Here's the drawing with two shaded views (mm, measured from the low corner). I have some questions. A direction names the side the tool comes from. Give positions to 0.01 mm unless a question says otherwise; leave off trailing zeros. Write each loop counter-clockwise with the first axis right and the second up, starting at its lowest first coordinate (ties: lowest second). Pieces come first, ordered by that corner, then holes. Notation, with made-up numbers: (-23, 8.25) - (26, 8.25) arc R22 cw to (26, 31.25) - close; hole circle Ø7 at (0.5, -33.5). An arc over 180 degrees is marked (long way). Write item = value, one per line.
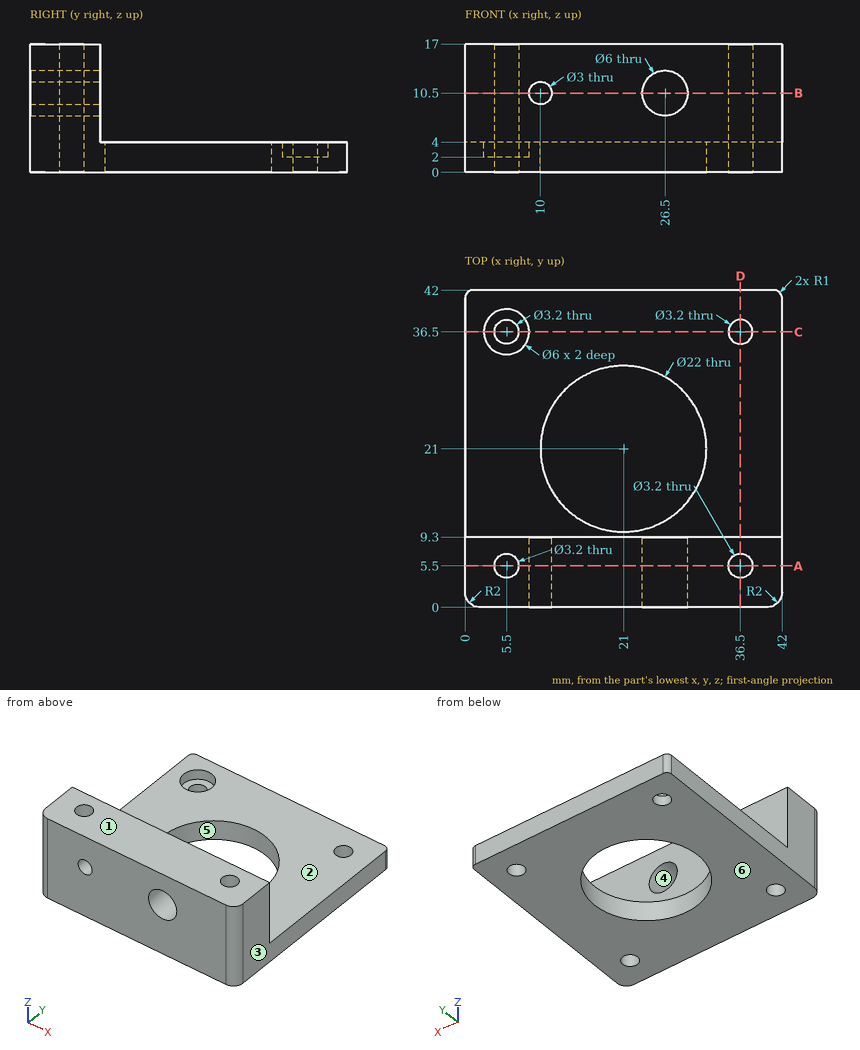
1. For pin 1 (2.5 mm diameter, centred on x = 10, z = 10.5, fed in from -Y); pin 2 (2 mm diameter, centred on x = 31, y = 31, fed in from +Z); pin 3 (4 mm diameter, centred on x = 26.5, z = 7.5, fed in from +Y); pin 4 (5 mm diameter, centred on x = 5.5, y = 36.5, fed in from +Z), each with a flat end and sliding along its axis, tell me the tip position at first contact or that it passes through.
Filled sheet:
pin_1 = through
pin_2 = 4
pin_3 = 9.3
pin_4 = 2
2. Thinking about a two-plate mould opening in X: for the marked faces 3, 4, 5 and 6, which applies, pulls with the +X half, pulls with the -X half, needs draft (parallel to the pull), parting line crosses it, or undercut?
Filled sheet:
face_3 = pulls with the +X half
face_4 = undercut
face_5 = undercut
face_6 = needs draft
3. If we section it at C-C, the plane y = 36.5: Please give me the cut outline in (x, z).
Filled sheet:
outline = (0, 0) - (3.9, 0) - (3.9, 2) - (2.5, 2) - (2.5, 4) - (0, 4) - close; (7.1, 0) - (34.9, 0) - (34.9, 4) - (8.5, 4) - (8.5, 2) - (7.1, 2) - close; (38.1, 0) - (42, 0) - (42, 4) - (38.1, 4) - close
4. Which directions (+Z, -Z, +X, -X, +Y, -Y) give clear straight access to the entire face, cutting with the end or side of a thin tool? Please do the marked faces 1 and 2.
Filled sheet:
face_1 = +Z, +X, -X, +Y, -Y
face_2 = +Z, +X, -X, +Y
5. If we section it at A-A, the plane y = 5.5: Please give me the cut outline in (x, z).
Filled sheet:
outline = (0, 0) - (3.9, 0) - (3.9, 17) - (0, 17) - close; (7.1, 0) - (34.9, 0) - (34.9, 17) - (7.1, 17) - close; (38.1, 0) - (42, 0) - (42, 17) - (38.1, 17) - close; hole circle Ø3 at (10, 10.5); hole circle Ø6 at (26.5, 10.5)
6. If we section it at D-D, the plane x = 36.5: Please give me the cut outline in (y, z), and give its area (3 significant figures).
Filled sheet:
outline = (0, 0) - (3.9, 0) - (3.9, 17) - (0, 17) - close; (7.1, 0) - (34.9, 0) - (34.9, 4) - (9.3, 4) - (9.3, 17) - (7.1, 17) - close; (38.1, 0) - (42, 0) - (42, 4) - (38.1, 4) - close
area = 222 mm2
7. I need wall thicknesses on line 1 (Y direction, x = 5.5, z = 1.4); line 2 (Y direction, x = 26.5, z = 5.5); line 3 (X direction, y = 8, z = 10.25). Which ranges of each line are inside material? Lowest first, please.
Filled sheet:
line_1 = 0 to 3.9, 7.1 to 34.9, 38.1 to 42
line_2 = 0 to 9.3
line_3 = 0 to 8.52, 11.48 to 23.51, 29.49 to 42
8. If we section it at B-B, the plane z = 10.5: Please give me the cut outline in (x, y).
Filled sheet:
outline = (0, 2) arc R2 ccw to (2, 0) - (8.5, 0) - (8.5, 9.3) - (0, 9.3) - close; (11.5, 0) - (23.5, 0) - (23.5, 9.3) - (11.5, 9.3) - close; (29.5, 0) - (40, 0) arc R2 ccw to (42, 2) - (42, 9.3) - (29.5, 9.3) - close; hole circle Ø3.2 at (5.5, 5.5); hole circle Ø3.2 at (36.5, 5.5)
